from build123d import *

# Parameters (mm, degrees)
F3_R     = 2.75
F4_DEPTH = 6


# Not quite as in the source:
# - a fillet or chamfer that OpenCascade refuses, or shapes differently, is made with other operations: its cross-section is extruded or revolved along the edge and cut away or added


with BuildPart() as f1:
    # F0 (on Front) → F1 (revolve)
    with BuildSketch(Plane.XZ):
        with BuildLine():
            Line((-4, 6), (-4, 0))
            Line((-4, 0), (0, 0))
            Line((0, 0), (0, 8.9428911653))
            ThreePointArc((0, 8.9428911653), (-5.525338883, 9.2077757466), (-11, 10))
            Line((-11, 10), (-11, 6))
            Line((-11, 6), (-4, 6))
        make_face()
    revolve(axis=Axis((0, 0, 4.4714455826), (0, 0, 1)))

    # F2: chamfer of 1 on 1 edges, made by hand

    # F2_s1 → F2_t2 (revolve, cut)
    with BuildSketch(Plane.XZ):
        with BuildLine():
            Line((-11.0306422703, 8.9829547915), (-10.0014779949, 9.846492555))
            Line((-10.0014779949, 9.846492555), (-9.9980042766, 9.866188577))
            ThreePointArc((-9.9980042766, 9.866188577), (-10.5002890164, 9.9256794224), (-10.996191144, 10.0196339659))
            Line((-10.996191144, 10.0196339659), (-11.02, 10))
            ThreePointArc((-11.02, 10), (-11.02, 9.4914773958), (-11.0506422703, 8.9829547915))
            Line((-11.0506422703, 8.9829547915), (-11.0306422703, 8.9829547915))
        make_face()
    revolve(axis=Axis((0, 0, 10), (0, 0, 1)), mode=Mode.SUBTRACT)

    # F3 (on face) → F4 (cut)
    with BuildSketch(Plane(origin=(0, 0, 0), x_dir=(1, 0, 0), z_dir=(0, 0, -1))):
        Circle(F3_R)
    extrude(amount=-F4_DEPTH, mode=Mode.SUBTRACT)


solid = f1.part
For this review, take the finished solid that the model builds, in its own axes (mm). A direction names the side the tool comes from. Round coordinates to 2 decimals unless told otherwise and drop trailing zeros. Write each loop counter-clockwise with the first axis right and the second up, starting at its lowest first coordinate (ties: lowest second). Pieces come first, ordered by that corner, then holes. Notation, with made-up numbers: (18, 74) - (62, 74) arc R26 cw to (62, 99) - close; hole circle Ø11 at (3.25, -28). An arc over 180 degrees is marked (long way). Write item = value, one per line. Start each with the question number.
1. Wall thickness on L1, parallel to X at y = 0, z = 4.55; L2, parallel to Z at x = -2.75, y = -0.75: over which ranges is each line inside the solid? List them lowest first.
2. Consider section C-C on z = 5.25. State the section outline as (x, y) points.
3. Draft analysis for pull direction Y (two halves, no side actions). For faces 3 (the face through (-0.596, 2.685, 2.958)), 4 (the face through (0, 5, 6)), 5 (the face through (2.38, 10.74, 7.48)), state which applies: released by +Y, released by -Y, zero draft, split by the parting line, or undercut.
4. For faces 1 (the face through (-3, -1, 0)), 2 (the face through (0.867, 3.905, 2.958)), list the 3-axis set-ups (+Z, -Z, +X, -X, +Y, -Y) from which the entire face can be reached by the end or side of a thin tool; tool diameter is ignored.
5. Consider section A-A on x = 0. State the section outline as (y, z) points, plus the area to 3 significant figures.
6. For pin 1 Ø3 at (x, y) = (0.5, -7) entering from +Z; pin 2 Ø6 at (x, y) = (-1, 3) entering from +Z; pin 3 Ø2 at (x, z) = (3, 8.5) entering from -Y, all flat-tipped, find the tip position at first contact; note any pin that passes through.
7. Consider section D-D on z = 8.5. State the section outline as (x, y) points.
Evaluation:
q1.L1 = -4 to -2.75, 2.75 to 4
q1.L2 = 0 to 9.01
q2.outline = circle Ø8 at (0, 0); hole circle Ø5.5 at (0, 0)
q3.face_3 = undercut
q3.face_4 = zero draft
q3.face_5 = split by the parting line
q4.face_1 = -Z, +X, -X, +Y, -Y
q4.face_2 = -Z
q5.outline = (-11, 6) - (-4, 6) - (-4, 0) - (-2.75, 0) - (-2.75, 6) - (2.75, 6) - (2.75, 0) - (4, 0) - (4, 6) - (11, 6) - (11, 9.01) - (10.03, 9.82) arc R57.76 cw to (-10.03, 9.82) - (-11, 9.01) - close
q5.area = 86.5 mm2
q6.pin_1 = 9.57
q6.pin_2 = 9.27
q6.pin_3 = -10.82
q7.outline = circle Ø22 at (0, 0)
